Check sheet for the modelled part. Datum: model origin and axes. Units: mm. A direction names the side the tool comes from. Round coordinates to 2 decimals unless told otherwise and drop trailing zeros. Write each loop counter-clockwise with the first axis right and the second up, starting at its lowest first coordinate (ties: lowest second). Pieces come first, ordered by that corner, then holes. Notation, with made-up numbers: (46.25, -16) -> (50.25, -16) arc R22 cw to (50.25, 9) -> close; hole circle Ø8 at (45.5, 46.25). An arc over 180 degrees is marked (long way). Put each result on its own line as item: value. Start each with the question number.
Autodesk Inventor part; units mm, degrees
ref_plane "YZ Plane" through (0, 0, 0) normal (1, 0, 0) x (0, 1, 0)
ref_plane "XZ Plane" through (0, 0, 0) normal (0, 1, 0) x (-1, 0, 0)
ref_plane "XY Plane" through (0, 0, 0) normal (0, 0, 1) x (1, 0, 0)
sketch "Sketch1" plane through (0, 0, 0) normal (0, 0, 1) x (1, 0, 0)
  line L0 (-54.7, 0) -> (-49, 0)
  line L1 (-50.7, -25) -> (-52.7, -25)
  line L2 (-54.7, -23) -> (-54.7, 0)
  line L3 (-47, 20) -> (-50, 20)
  line L4 (-50, 20) -> (-50, 58)
  line L5 (-48, 60) -> (-47, 60)
  line L6 (-47, 60) -> (-47, 20)
  line L7 (-54.7, 0) -> (-65.3724, 0)
  line L8 (-65.3724, 0) -> (-50, 20)
  line L9 (-47, 20) -> (-47, 2)
  arc A0 (-48, 60) -> (-50, 58) centre (-48, 58) ccw
  arc A1 (-54.7, -23) -> (-52.7, -25) centre (-52.7, -23) ccw
  line L10 (0, -42.5799) -> (0, 77.5799)
  line L11 (-50.7, -25) -> (-50.7, 0)
  arc A2 (-49, 0) -> (-47, 2) centre (-49, 2) ccw
  point P0 (0, 0)
  point P1 (-47, 0)
  point P2 (-54.7, -25)
  point P3 (-50, 60)
  point P4 (-51.85, 0)
  dimension "d7" = 40
  dimension "d10" = 2
  dimension "d12" = 20
  dimension "d20" = 50
  dimension "d21" = 54.7
  dimension "d22" = 3
  dimension "d23" = 2
  dimension "d24" = 4
revolve "Revolution1" add sketch "Sketch1" angle 360 about axis through (0, -10, 0) along (0, 1, 0)
sketch "Sketch2" plane through (0, -25, 0) normal (0, -1, 0) x (1, 0, 0)
  line L0 (1.5, 45.7) -> (-1.5, 45.7)
  line L1 (-1.5, 45.7) -> (-1.5, 55.7)
  line L2 (-1.5, 55.7) -> (1.5, 55.7)
  line L3 (1.5, 55.7) -> (1.5, 45.7)
  circle A0 centre (0, 0) radius 50.7
  line L4 (1.5, 45.7) -> (-1.5, 55.7) construction
  line L5 (-1.5, 45.7) -> (1.5, 55.7) construction
  point P0 (0, 50.7)
  dimension "d13" = 3
  dimension "d14" = 10
extrude "Extrusion1" cut sketch "Sketch2" against normal blind 25 contours L0 L1 A0 L3 | A0 L1 L2 L3 picked at (0.1667, 47.3658)
pattern_circular "Circular Pattern1" count 6 over 360 about axis through (0, -10, 0) along (0, 1, 0) of "Extrusion1"
properties part number "top-ventilation-tube-adapter-109.6mmID-to-100mmID"
1. Draft check along Z on faces 5 (the flat face through (-44.895, -12.675, 27.652)), 6 (the flat face through (44.895, -12.675, -27.652)), 7 (the cylindrical face through (-27.02, -11.34, -47.56)), 8 (the flat face through (26, -25, 44)). Enter one of: released by +Z, released by -Z, zero draft, split by the parting line, or undercut.
2. Material ranges on L1, parallel to Z at x = 0, y = 28; L2, parallel to X at y = 6.5, z = 25; L3, parallel to Z at x = 0, y = 14, recorded low to high. Write a range as [from, to].
3. Section check B-B, the plane y = 36.5. Enter the section's corners in (x, z), then the cut area to 3 significant figures.
4. Section check A-A, the plane z = 0. Enter the section's corners in (x, y), then the cut area to 3 significant figures.
5. Access from +Z, -Z, +X, -X, +Y, -Y to the whole of each face (thin tool, end or side, straight path). Record for faces 1 (the cylindrical face through (27.68, -11.34, -47.18)), 2 (the cylindrical face through (-25.653, -12.325, 43.731)), 3 (the flat face through (44.847, -12.675, 27.624)), 4 (the cylindrical face through (-27.68, -11.34, 47.18)).
6. Gauge pin test, flat ends, axial feed: P1, Ø4, axis at x = -33, y = 19.5, coming from the +Z side; P2, Ø1, axis at x = -37, y = 33.5, coming from the +Z side; P3, Ø10, axis at y = 3.5, z = 35, coming from the -X side. Record the tip position at first contact, or that the pin passes through.
Reply:
1. face 5: undercut
1. face 6: undercut
1. face 7: released by -Z
1. face 8: zero draft
2. L1: z = [-50, -47], [47, 50]
2. L2: x = [-54.96, -39.8], [39.8, 54.96]
2. L3: z = [-54.61, -47], [47, 54.61]
3. outline: circle Ø100 at (0, 0); hole circle Ø94 at (0, 0)
3. area: 914 mm2
4. outline: (-65.37, 0) -> (-54.7, 0) -> (-54.7, -23) arc R2 ccw to (-52.7, -25) -> (-50.7, -25) -> (-50.7, 0) -> (-49, 0) arc R2 ccw to (-47, 2) -> (-47, 60) -> (-48, 60) arc R2 ccw to (-50, 58) -> (-50, 20) -> close; (47, 2) arc R2 ccw to (49, 0) -> (50.7, 0) -> (50.7, -25) -> (52.7, -25) arc R2 ccw to (54.7, -23) -> (54.7, 0) -> (65.37, 0) -> (50, 20) -> (50, 58) arc R2 ccw to (48, 60) -> (47, 60) -> close
4. area: 862 mm2
5. face 1: -Z, +X, -Y
5. face 2: -Y
5. face 3: +X, -Y
5. face 4: +Z, -X, -Y
6. P1: stops at z = 40.66
6. P2: stops at z = 34.17
6. P3: stops at x = -57.32
